```python
from build123d import *

# Parameters (mm, degrees)
SKETCH_1_W          = 60
SKETCH_1_H          = 50
SKETCH_1_R          = 15
EXTRUDE_5_DEPTH     = 5
SKETCH_4_W          = 60
SKETCH_4_H          = 50
SKETCH_4_R          = 5.5
EXTRUDE_6_DEPTH     = 5
SKETCH_5_R          = 1.6
CUT_EXTRUDE_1_DEPTH = 10
SKETCH_6_W          = 60
SKETCH_6_H          = 10
EXTRUDE_7_DEPTH     = 7
FILLET_3_R          = 10
FILLET_5_R          = 10
FILLET_6_R          = 5
FILLET_7_R          = 5
SKETCH_7_W          = 62.929868023
SKETCH_7_H          = 59.60365164
CUT_EXTRUDE_2_DEPTH = 5
SKETCH_8_R          = 15
CUT_EXTRUDE_3_DEPTH = 2
SKETCH_9_R          = 15
CUT_EXTRUDE_4_DEPTH = 2
SKETCH_10_R         = 5.5
CUT_EXTRUDE_6_DEPTH = 44.965895874
SKETCH_11_R         = 5.5
EXTRUDE_8_DEPTH     = 3
EXTRUDE_START       = 2
EXTRUDE_9_DEPTH     = 2


with BuildPart() as part:
    # 草图1 → 凸台-拉伸5 (new body)
    with BuildSketch(Plane.XY):
        Rectangle(SKETCH_1_W, SKETCH_1_H)
        Circle(SKETCH_1_R, mode=Mode.SUBTRACT)
    extrude(amount=EXTRUDE_5_DEPTH)

    # 草图4 → 凸台-拉伸6 (add)
    with BuildSketch(Plane.XY.offset(5)):
        Rectangle(SKETCH_4_W, SKETCH_4_H)
        Circle(SKETCH_4_R, mode=Mode.SUBTRACT)
    extrude(amount=EXTRUDE_6_DEPTH)

    # 草图5 → 切除-拉伸1 (cut)
    with BuildSketch(Plane(origin=(0, 0, 0), x_dir=(-1, 0, 0), z_dir=(0, 0, -1))):
        with Locations((-20, 22)):
            Circle(SKETCH_5_R)
        with Locations((-25, -18)):
            Circle(SKETCH_5_R)
        with Locations((20, 22)):
            Circle(SKETCH_5_R)
        with Locations((25, -18)):
            Circle(SKETCH_5_R)
    extrude(amount=-CUT_EXTRUDE_1_DEPTH, mode=Mode.SUBTRACT)

    # 草图6 → 凸台-拉伸7 (add)
    with BuildSketch(Plane(origin=(0, 25, 0), x_dir=(1, 0, 0), z_dir=(0, 1, 0))):
        with Locations((0, -5)):
            Rectangle(SKETCH_6_W, SKETCH_6_H)
    extrude(amount=EXTRUDE_7_DEPTH)

    # 圆角3
    fillet_3_edges = [part.edges().sort_by_distance(p)[0] for p in [
        (-30, 32, 5),
    ]]
    fillet(fillet_3_edges, radius=FILLET_3_R)

    # 圆角5
    fillet_5_edges = [part.edges().sort_by_distance(p)[0] for p in [
        (30, 32, 5),
    ]]
    fillet(fillet_5_edges, radius=FILLET_5_R)

    # 圆角6
    fillet_6_edges = [part.edges().sort_by_distance(p)[0] for p in [
        (-30, -25, 5),
    ]]
    fillet(fillet_6_edges, radius=FILLET_6_R)

    # 圆角7
    fillet_7_edges = [part.edges().sort_by_distance(p)[0] for p in [
        (30, -25, 5),
    ]]
    fillet(fillet_7_edges, radius=FILLET_7_R)

    # 草图7 → 切除-拉伸2 (cut)
    with BuildSketch(Plane(origin=(0, 0, 0), x_dir=(-1, 0, 0), z_dir=(0, 0, -1))):
        with Locations((0.697432467, 2.50749995)):
            Rectangle(SKETCH_7_W, SKETCH_7_H)
    extrude(amount=-CUT_EXTRUDE_2_DEPTH, mode=Mode.SUBTRACT)

    # 草图8 → 切除-拉伸3 (cut)
    with BuildSketch(Plane(origin=(0, 0, 5), x_dir=(-1, 0, 0), z_dir=(0, 0, -1))):
        Circle(SKETCH_8_R)
    extrude(amount=-CUT_EXTRUDE_3_DEPTH, mode=Mode.SUBTRACT)

    # 草图9 → 切除-拉伸4 (cut)
    with BuildSketch(Plane(origin=(0, 0, 5), x_dir=(-1, 0, 0), z_dir=(0, 0, -1))):
        with Locations((0, 14)):
            Circle(SKETCH_9_R)
        Circle(SKETCH_9_R)
        with BuildLine():
            ThreePointArc((-13.266499161, 7), (-14.560176637, 10.394274513), (-15, 14))
            Line((-15, 14), (-15, 0))
            ThreePointArc((-15, 0), (-14.560176637, 3.605725487), (-13.266499161, 7))
        make_face()
        with BuildLine():
            Line((15, 0), (15, 14))
            ThreePointArc((15, 14), (14.560176637, 10.394274513), (13.266499161, 7))
            ThreePointArc((13.266499161, 7), (14.560176637, 3.605725487), (15, 0))
        make_face()
    extrude(amount=-CUT_EXTRUDE_4_DEPTH, mode=Mode.SUBTRACT)

    # 草图10 → 切除-拉伸6 (cut, through all)
    with BuildSketch(Plane(origin=(0, 0, 7), x_dir=(-1, 0, 0), z_dir=(0, 0, -1))):
        with Locations((0, 14)):
            Circle(SKETCH_10_R)
    extrude(amount=-CUT_EXTRUDE_6_DEPTH, mode=Mode.SUBTRACT)

    # 草图11 → 凸台-拉伸8 (add)
    with BuildSketch(Plane(origin=(0, 0, 7), x_dir=(-1, 0, 0), z_dir=(0, 0, -1))):
        Circle(SKETCH_11_R)
    extrude(amount=-EXTRUDE_8_DEPTH)

    # 草图12 → 凸台-拉伸9 (add)
    with BuildSketch(Plane(origin=(0, 0, 7), x_dir=(-1, 0, 0), z_dir=(0, 0, -1)).offset(EXTRUDE_START)):
        with BuildLine():
            ThreePointArc((-13.266499161, 7), (-14.560176637, 3.605725487), (-15, 0))
            ThreePointArc((-15, 0), (0, -15), (15, 0))
            ThreePointArc((15, 0), (14.560176637, 3.605725487), (13.266499161, 7))
            ThreePointArc((13.266499161, 7), (0, -1), (-13.266499161, 7))
        make_face()
        with BuildLine():
            ThreePointArc((-13.266499161, 7), (-14.560176637, 10.394274513), (-15, 14))
            Line((-15, 14), (-15, 0))
            ThreePointArc((-15, 0), (-14.560176637, 3.605725487), (-13.266499161, 7))
        make_face()
        with BuildLine():
            Line((15, 0), (15, 14))
            ThreePointArc((15, 14), (14.560176637, 10.394274513), (13.266499161, 7))
            ThreePointArc((13.266499161, 7), (14.560176637, 3.605725487), (15, 0))
        make_face()
    extrude(amount=-EXTRUDE_9_DEPTH)


solid = part.part
```
Design review of the part built by this model. Coordinates are the model's own, in mm. A direction names the side the tool comes from. Coordinates: 2 decimals unless noted, no trailing zeros. Loops run counter-clockwise (first coordinate to the right, second up) from the corner with the lowest first, then second, coordinate; pieces in that order, holes last.
Q1. We need section B-B on x = 0. State the section outline as (y, z) points.
Reported:
outline: (-25, 5) - (-1, 5) - (-1, 7) - (8.5, 7) - (8.5, 10) - (-25, 10) - close; (19.5, 7) - (29, 7) - (29, 5) - (32, 5) - (32, 10) - (19.5, 10) - close
Q2. We need section D-D on y = 1.5. State the section outline as (x, z) points, and give its area (3 significant figures).
Reported:
outline: (-30, 5) - (-8.29, 5) - (-8.29, 7) - (8.29, 7) - (8.29, 5) - (30, 5) - (30, 10) - (-30, 10) - close
area: 267 mm2
Q3. Tool access review of faces 5 (the face through (-18.82, 23.08, 7.46)), 6 (the face through (0, 8, 7)): name each direction out of +Z, -Z, +X, -X, +Y, -Y from which nothing blocks a thin tool from reaching the whole face with its end or side.
Reported:
face 5: +Z, -Z
face 6: -Z
Q4. The part is to be moulded in two halves that separate along Y. For faces 1 (the face through (0, -25, 7)), 2 (the face through (25.208, -16.414, 7.465)), 3 (the face through (-30, 1, 8)), 4 (the face through (26.99, 29.15, 7.46)), say which applies: +Y half, -Y half, draft (parallel to the pull), parting line (faces both ways), or undercut.
Reported:
face 1: -Y half
face 2: undercut
face 3: draft
face 4: +Y half
Q5. We need section C-C on y = 12. State the section outline as (x, z) points, and give its area (3 significant figures).
Reported:
outline: (-30, 5) - (-14.87, 5) - (-14.87, 7) - (-5.12, 7) - (-5.12, 10) - (-30, 10) - close; (5.12, 7) - (14.87, 7) - (14.87, 5) - (30, 5) - (30, 10) - (5.12, 10) - close
area: 210 mm2
Q6. We need section A-A on z = 6.25. State the section outline as (x, y) points, and give its area (3 significant figures).
Reported:
outline: (-30, -20) arc R5 ccw to (-25, -25) - (25, -25) arc R5 ccw to (30, -20) - (30, 22) arc R10 ccw to (20, 32) - (-20, 32) arc R10 ccw to (-30, 22) - close; hole circle Ø3.2 at (-25, -18); hole circle Ø3.2 at (-20, 22); hole circle Ø30 at (0, 14); hole circle Ø3.2 at (20, 22); hole circle Ø3.2 at (25, -18)
area: 2,630 mm2
Q7. To check wall thickness, follow line 1 (Y direction, x = 20, z = 7); line 2 (Z direction, x = -8, y = 1.5); line 3 (Y direction, x = -2.5, z = 7.4). State the ranges of each line that lie inside material, in increasing order.
Reported:
line 1: y = -25 to 20.4, 23.6 to 32
line 2: z = 7 to 10
line 3: y = -25 to 9.1, 18.9 to 32
Q8. For pin 1 (1.5 mm diameter, centred on x = 10, y = 24, fed in from -Z), flat-tipped, find the tip position at first contact; note if it passes through.
Reported:
pin 1: stops at z = 7
